Can you work these out from the drawing? Everything is in mm from the part's minimum corner. A direction names the side the tool comes from. Coordinates: 2 decimals unless noted, no trailing zeros. Order: outer loops, then holes, each group sorted by start corner. A loop starts at its lowest first (then second) coordinate and runs counter-clockwise, first axis right, second up. Notation, with made-up numbers: M -13.75,32 L 10.25,32 A24 ccw 10.25,43 Z; hole C -26,33 d9. An arc over 180 degrees is marked long. Answer as a JSON object with one key per item and string values.
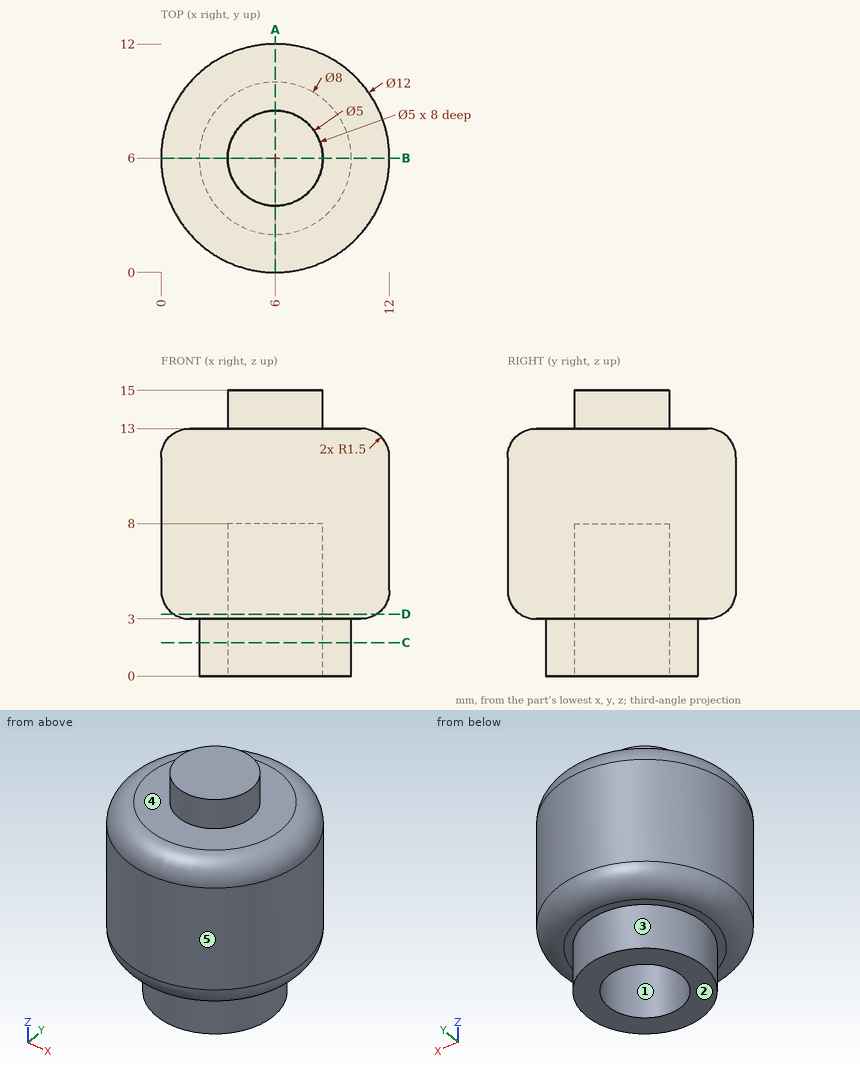
Item 1: Which directions (+Z, -Z, +X, -X, +Y, -Y) give clear straight access to the entire face, cutting with the end or side of a thin tool? Please do the marked faces 4 and 5.
Answers follow:
{"face 4": "+Z", "face 5": "+Z, -Z"}
Item 2: Please list where these lines run through material, in increasing order: line 1 (Z direction, x = 4, y = 4); line 2 (Y direction, x = 6, z = 4.5); line 3 (Z direction, x = 7.75, y = 7.25).
Answers follow:
{"line 1": "z = 0 to 13", "line 2": "y = 0 to 3.5, 8.5 to 12", "line 3": "z = 8 to 15"}
Item 3: I want a section at D-D, the plane z = 3.25. Write out the boundary of the cut face in (x, y).
Answers follow:
{"outline": "C 6,6 d10.66; hole C 6,6 d5"}
Item 4: If we mould it in two halves opening along Y, with no side actions, what happens to the marked faces 1, 2 and 3? For each: pulls with the +Y half, pulls with the -Y half, needs draft (parallel to the pull), parting line crosses it, or undercut.
Answers follow:
{"face 1": "undercut", "face 2": "needs draft", "face 3": "parting line crosses it"}
Item 5: I'm going to push flat-ended pins straight in: pin 1 (3 mm diameter, centred on x = 2, y = 1, fed in from -Z); pin 2 (1 mm diameter, centred on x = 9, y = 4, fed in from +Z); pin 3 (3 mm diameter, centred on y = 4, z = 9, fed in from +X). Where does each tip first touch, or does it pass through?
Answers follow:
{"pin 1": "stops at z = 3.06", "pin 2": "stops at z = 13", "pin 3": "stops at x = 11.98"}
Item 6: I want a section at A-A, the plane x = 6. Write out the boundary of the cut face in (y, z).
Answers follow:
{"outline": "M 0,4.5 A1.5 ccw 1.5,3 L 2,3 L 2,0 L 3.5,0 L 3.5,8 L 8.5,8 L 8.5,0 L 10,0 L 10,3 L 10.5,3 A1.5 ccw 12,4.5 L 12,11.5 A1.5 ccw 10.5,13 L 8.5,13 L 8.5,15 L 3.5,15 L 3.5,13 L 1.5,13 A1.5 ccw 0,11.5 Z"}
Item 7: I want a section at C-C, the plane z = 1.75. Write out the boundary of the cut face in (x, y).
Answers follow:
{"outline": "C 6,6 d8; hole C 6,6 d5"}
